Here's how the part is built. I have some questions about the finished solid (model axes, mm). Face numbers are marked on the shaded views. A direction names the side the tool comes from. Coordinates: 2 decimals unless noted, no trailing zeros. Loops run counter-clockwise (first coordinate to the right, second up) from the corner with the lowest first, then second, coordinate; pieces in that order, holes last. Notation, with made-up numbers: (-2, 42) -> (56, 42) arc R22 cw to (56, 67) -> close; hole circle Ø9 at (-20, 80). An arc over 180 degrees is marked (long way). Answer as a JSON object with one key per item and string values. Group by question number.
1) I want a section at A-A (z = 8.5). Write out the boundary of the cut face in (x, y), then the cut area to 3 significant figures.
2) I'm going to push flat-ended pins straight in: pin 1 (2 mm diameter, centred on y = -16, z = 8, fed in from +X); pin 2 (5.5 mm diameter, centred on y = 3, z = 7.5, fed in from -X); pin 3 (4 mm diameter, centred on x = -3.5, z = 3, fed in from +Y); pin 4 (8 mm diameter, centred on x = 4, y = -8, fed in from +Z). Where does each tip first touch, or does it pass through?
3) If we mould it in two halves opening along X, with no side actions, what happens to the marked faces 1, 2 and 3? For each: +X half, -X half, draft (parallel to the pull), parting line (faces both ways), or undercut.
4) I need wall thicknesses on probe 1 along X at (y, z) = (24.5, 9.5); probe 2 along X at (y, z) = (-4, 13.75); probe 3 along Y at (x, z) = (7.5, 12.5). Which ranges of each line are inside material? Lowest first, please. Write a range as [from, to].
5) Which directions (+Z, -Z, +X, -X, +Y, -Y) give clear straight access to the entire face, cutting with the end or side of a thin tool? Please do the marked faces 4, 5 and 6.
6) I want a section at C-C (x = -4). Write out the boundary of the cut face in (y, z).
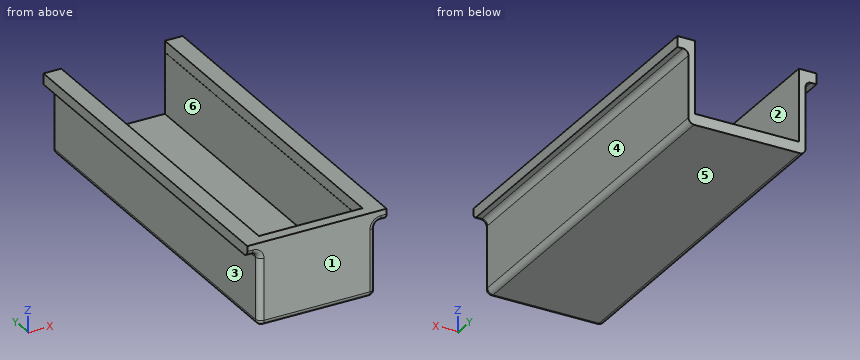
```python
from build123d import *

# Parameters (mm, degrees)
ESQUISSE1_W                  = 25
ESQUISSE1_H                  = 65
BOSS_EXTRU_1_DEPTH           = 15
ENL_V_MAT_EXTRU_1_DEPTH      = 68.869359802
ENL_V_MAT_EXTRU_1_DEPTH_BACK = 68.869359802
ESQUISSE2_W                  = 1.99730465
ESQUISSE2_H                  = 13.055396478
ESQUISSE3_W                  = 18.6
ESQUISSE3_H                  = 10.964826829
ENL_V_MAT_EXTRU_2_DEPTH      = 63
ESQUISSE4_W                  = 18.610580781
ESQUISSE4_H                  = 2.037454763
ENL_V_MAT_EXTRU_3_DEPTH      = 63
CONG_1_R                     = 1


with BuildPart() as part:
    # Esquisse1 → Boss.-Extru.1 (new body)
    with BuildSketch(Plane.XY):
        Rectangle(ESQUISSE1_W, ESQUISSE1_H)
    extrude(amount=BOSS_EXTRU_1_DEPTH)

    # Esquisse2 → Enlèv. mat.-Extru.1 (cut, two sides: drawn at the far end of the back side and taken through both)
    with BuildSketch(Plane(origin=(0, 32.5, 0), x_dir=(1, 0, 0), z_dir=(0, 1, 0)).offset(-ENL_V_MAT_EXTRU_1_DEPTH_BACK)):
        with Locations((11.501347675, -6.527698239)):
            Rectangle(ESQUISSE2_W, ESQUISSE2_H)
        with Locations((-11.501347675, -6.527698239)):
            Rectangle(ESQUISSE2_W, ESQUISSE2_H)
    extrude(amount=ENL_V_MAT_EXTRU_1_DEPTH + ENL_V_MAT_EXTRU_1_DEPTH_BACK, mode=Mode.SUBTRACT)

    # Esquisse3 → Enlèv. mat.-Extru.2 (cut)
    with BuildSketch(Plane(origin=(0, 32.5, 0), x_dir=(1, 0, 0), z_dir=(0, 1, 0))):
        with Locations((0, -7.480131823)):
            Rectangle(ESQUISSE3_W, ESQUISSE3_H)
    extrude(amount=-ENL_V_MAT_EXTRU_2_DEPTH, mode=Mode.SUBTRACT)

    # Esquisse4 → Enlèv. mat.-Extru.3 (cut)
    with BuildSketch(Plane(origin=(0, 32.5, 0), x_dir=(1, 0, 0), z_dir=(0, 1, 0))):
        with Locations((0.00529039, -13.981272619)):
            Rectangle(ESQUISSE4_W, ESQUISSE4_H)
    extrude(amount=-ENL_V_MAT_EXTRU_3_DEPTH, mode=Mode.SUBTRACT)

    # Congé1
    cong_1_edges = [part.edges().sort_by_distance(p)[0] for p in [
        (0, -32.5, 0),
        (-10.50269535, 0, 13.055396478),
        (-11.501347675, -32.5, 13.055396478),
        (-10.50269535, 0, 0),
        (-10.50269535, -32.5, 6.527698239),
        (10.50269535, 0, 0),
        (11.501347675, -32.5, 13.055396478),
        (10.50269535, 0, 13.055396478),
        (10.50269535, -32.5, 6.527698239),
    ]]
    fillet(cong_1_edges, radius=CONG_1_R)


solid = part.part
```
Determined:
{
 "1": {"outline": "(-10.5, -31.5) arc R1 ccw to (-9.5, -32.5) -> (9.5, -32.5) arc R1 ccw to (10.5, -31.5) -> (10.5, 32.5) -> (9.3, 32.5) -> (9.3, -30.5) -> (-9.3, -30.5) -> (-9.3, 32.5) -> (-10.5, 32.5) -> close", "area": "193 mm^2"},
 "2": {"pin 1": "x = 10.5", "pin 2": "x = -10.5", "pin 3": "y = 32.5", "pin 4": "z = 2"},
 "3": {"face 1": "draft", "face 2": "undercut", "face 3": "-X half"},
 "4": {"probe 1": "[-10.5, -9.3], [9.3, 10.5]", "probe 2": "[-12.5, -9.3], [9.31, 12.5]", "probe 3": "[-32.5, -30.5]"},
 "5": {"face 4": "-Z, +X, +Y, -Y", "face 5": "-Z, +X, -X, +Y, -Y", "face 6": "+Z, +Y"},
 "6": {"outline": "(-32.5, 1) arc R1 ccw to (-31.5, 0) -> (32.5, 0) -> (32.5, 2) -> (-30.5, 2) -> (-30.5, 15) -> (-32.5, 15) -> close"}
}
